The model under review builds one solid part; all positions refer to its coordinate system, in mm. A direction names the side the tool comes from. Give positions to 0.01 mm unless a question says otherwise; leave off trailing zeros. Order: outer loops, then holes, each group sorted by start corner. A loop starts at its lowest first (then second) coordinate and runs counter-clockwise, first axis right, second up. Notation, with made-up numbers: (63, 13.5) - (78, 13.5) arc R31 cw to (78, 42.5) - close; hole circle Ø7 at (23, -12.75). An arc over 180 degrees is marked (long way). Put each result on its own line as item: value.
```python
from build123d import *

# Parameters (mm, degrees)
F0_R     = 4
F1_DEPTH = 5
F2_DEPTH = 25
F3_SIZE  = 1


with BuildPart() as f1:
    # F0 (on Front) → F1 (new body)
    with BuildSketch(Plane.XZ):
        with BuildLine():
            ThreePointArc((5.6291651023, -3.2500000386), (6.2785178651, -1.6823238147), (6.5, 0))
            ThreePointArc((6.5, 0), (6.2785178797, 1.6823237603), (5.6291651586, 3.2499999411))
            ThreePointArc((5.6291651586, 3.2499999411), (3.2500000295, 5.6291651076), (0, 6.5))
            ThreePointArc((0, 6.5), (-3.2499999993, 5.629165125), (-5.6291651238, 3.2500000014))
            ThreePointArc((-5.6291651238, 3.2500000014), (-6.5, -6.45e-08), (-5.6291650593, -3.2500001131))
            ThreePointArc((-5.6291650593, -3.2500001131), (-3.2499999434, -5.6291651573), (0, -6.5))
            ThreePointArc((0, -6.5), (3.2499999807, -5.6291651357), (5.6291651023, -3.2500000386))
        make_face()
        Circle(F0_R, mode=Mode.SUBTRACT)
        Circle(F0_R)
        with BuildLine():
            ThreePointArc((5.6291651586, 3.2499999411), (6.2785178797, 1.6823237603), (6.5, 0))
            ThreePointArc((6.5, 0), (6.2785178651, -1.6823238147), (5.6291651023, -3.2500000386))
            Line((5.6291651023, -3.2500000386), (7.5055534995, 0))
            Line((7.5055534995, 0), (5.6291651586, 3.2499999411))
        make_face()
        with BuildLine():
            Line((3.7527767497, -6.5), (5.6291651023, -3.2500000386))
            ThreePointArc((5.6291651023, -3.2500000386), (3.2499999807, -5.6291651357), (0, -6.5))
            Line((0, -6.5), (3.7527767497, -6.5))
        make_face()
        with BuildLine():
            ThreePointArc((0, 6.5), (3.2500000295, 5.6291651076), (5.6291651586, 3.2499999411))
            Line((5.6291651586, 3.2499999411), (3.7527767497, 6.5))
            Line((3.7527767497, 6.5), (0, 6.5))
        make_face()
        with BuildLine():
            ThreePointArc((-5.6291651238, 3.2500000014), (-3.2499999993, 5.629165125), (0, 6.5))
            Line((0, 6.5), (-3.7527767497, 6.5))
            Line((-3.7527767497, 6.5), (-5.6291651238, 3.2500000014))
        make_face()
        with BuildLine():
            ThreePointArc((-5.6291650593, -3.2500001131), (-6.5, -6.45e-08), (-5.6291651238, 3.2500000014))
            Line((-5.6291651238, 3.2500000014), (-7.5055534995, 0))
            Line((-7.5055534995, 0), (-5.6291650593, -3.2500001131))
        make_face()
        with BuildLine():
            Line((-3.7527767497, -6.5), (0, -6.5))
            ThreePointArc((0, -6.5), (-3.2499999434, -5.6291651573), (-5.6291650593, -3.2500001131))
            Line((-5.6291650593, -3.2500001131), (-3.7527767497, -6.5))
        make_face()
    extrude(amount=F1_DEPTH)

    # F0 (on Front) → F2 (join)
    with BuildSketch(Plane.XZ):
        Circle(F0_R)
    extrude(amount=-F2_DEPTH)

    # F3
    f3_edges = [f1.edges().sort_by_distance(p)[0] for p in [
        (-4, 25, 0),
    ]]
    chamfer(f3_edges, length=F3_SIZE)

    # F4 (on Right) → F5 (revolve, cut)
    with BuildSketch(Plane.YZ):
        Polygon((-7.5355339059, 9.5203164965), (-7.5355339059, 4.1202170542), (-4, 7.6557509601), (-2.5, 7.6557509601), (-1, 7.6557509601), (2.5355339059, 4.1202170542), (2.5379077522, 9.5203164965), align=None)
    revolve(axis=Axis((0, 10, 0), (0, 1, 0)), mode=Mode.SUBTRACT)


solid = f1.part
```
(1) Wall thickness on L1, parallel to Y at x = 3.5, z = -3.25; L2, parallel to Z at x = 0, y = 15; L3, parallel to X at y = 2, z = 0.25: over which ranges is each line inside the solid? List them lowest first.
The answers:
L1: -5 to 0
L2: -4 to 4
L3: -3.99 to 3.99
(2) Clearance check with flat-ended pins moving along their axes: pin 1 Ø3 at (y, z) = (20.5, 0.5) entering from -X; pin 2 Ø2 at (y, z) = (18, 2.5) entering from -X; pin 3 Ø3 at (y, z) = (20.5, -4) entering from +X; pin 4 Ø1 at (x, z) = (-6, -5) entering from +Y. State where each tip first meets the part, or that it passes through.
The answers:
pin 1: x = -4
pin 2: x = -3.71
pin 3: x = 3.12
pin 4: through
(3) Take a section at A-A, the plane x = 0. Write out the cut boundary in (y, z).
The answers:
outline: (-5, -6.5) - (0, -6.5) - (0, -4) - (24, -4) - (25, -3) - (25, 3) - (24, 4) - (0, 4) - (0, 6.5) - (-5, 6.5) - close
(4) Take a section at B-B, the plane y = 8. Write out the cut boundary in (x, z).
The answers:
outline: circle Ø8 at (0, 0)
(5) For faces 1 (the cylindrical face through (-0.867, 11.832, -3.905)), 2 (the flat face through (0, -2, 6.5)), list the 3-axis set-ups (+Z, -Z, +X, -X, +Y, -Y) from which the entire face can be reached by the end or side of a thin tool; tool diameter is ignored.
The answers:
face 1: +Y
face 2: +Z, +X, -X, +Y, -Y
